Input: part model. Units: mm. Frame: model coordinates. A direction names the side the tool comes from. Round coordinates to 2 decimals unless told otherwise and drop trailing zeros. Loops run counter-clockwise (first coordinate to the right, second up) from the corner with the lowest first, then second, coordinate; pieces in that order, holes last.
1) Draft query along X for faces 1 (the face through (25, -26, 3)), 2 (the face through (-0.54, 52.33, 2.54)), 3 (the face through (0, -100, 20)). Return one class per face: pulls with the +X half, pulls with the -X half, needs draft (parallel to the pull), parting line crosses it, or undercut.
2) Section B-B, the plane y = 54.77. Return loops of the section in (x, z), and give its area (3 significant figures).
3) Access query for faces 4 (the face through (-25, -27, 4)), 5 (the face through (0, -9, 5)). Directions: +Z, -Z, +X, -X, +Y, -Y. A direction counts if a zero-diameter tool reaches every point of the face in a straight line with its end or side. Return the directions, or none.
4) Section D-D, the plane x = -19. Return loops of the section in (y, z).
5) First-contact query: pin 1 (9 mm diameter, centred on x = -8.5, z = 14.5, fed in from +Y); pin 2 (25 mm diameter, centred on x = -3, y = -45.5, fed in from +Z). Flat tips, straight axial feed; report the tip coordinate or a pass-through.
6) Section A-A, the plane x = 0. Return loops of the section in (y, z).
7) Ray query, line 1 along Y through (x, z) = (0, 3); line 2 along X through (y, z) = (42.6, 1.2); line 3 along Z through (x, y) = (-2, -86.5). Return the intervals inside material, ascending.
8) Section C-C, the plane z = 9. Return loops of the section in (x, y).
Autodesk Inventor part; units mm, degrees
ref_plane "YZ Plane" through (0, 0, 0) normal (1, 0, 0) x (0, 1, 0)
ref_plane "XZ Plane" through (0, 0, 0) normal (0, 1, 0) x (-1, 0, 0)
ref_plane "XY Plane" through (0, 0, 0) normal (0, 0, 1) x (1, 0, 0)
sketch "Sketch1" plane through (0, 0, 0) normal (0, 0, 1) x (1, 0, 0)
  line L0 (-25, -110) -> (-25, 110)
  line L1 (-25, 110) -> (25, 110)
  line L2 (25, 110) -> (25, -110)
  line L3 (25, -110) -> (-25, -110)
  line L4 (-25, -110) -> (25, 110) construction
  line L5 (-25, 110) -> (25, -110) construction
  line L6 (-25, -110) -> (-25, -105)
  line L7 (-25, -105) -> (25, -105)
  point P0 (0, 0)
  dimension "d0" = 220
  dimension "d1" = 50
  dimension "d2" = 5
extrude "Extrusion1" add sketch "Sketch1" along normal blind 5 contours L0 L1 L2 L7
sketch "Sketch2" plane through (0, 0, 5) normal (0, 0, 1) x (1, 0, 0)
  line L0 (-25, 110) -> (-25, -105)
  line L1 (-25, -105) -> (-25, -100)
  line L2 (-25, -100) -> (25, -100)
  line L3 (25, -105) -> (25, 110)
  line L4 (25, -100) -> (25, -105)
  line L5 (-25, -105) -> (25, -105)
  line L6 (-25, -105) -> (25, -105)
  point P0 (0, 0)
  dimension "d5" = 5
extrude "Extrusion2" add sketch "Sketch2" along normal blind 30
sketch "Sketch3" plane through (0, 0, 5) normal (0, 0, 1) x (1, 0, 0)
  line L0 (25, 110) -> (-25, 110)
  line L1 (0, 110) -> (-5, 110)
  line L2 (-5, 110) -> (5, 110)
  arc A0 (-5, 110) -> (5, 110) centre (0, 110) ccw
  point P0 (0, 0)
  dimension "d8" = 5
  dimension "d9" = 10
  dimension "d10" = 5
extrude "Extrusion3" cut sketch "Sketch3" against normal blind 30
ref_plane "Work Plane1" through (0, -105, 0) normal (1, 0, 0) x (0, 0, -1)
sketch "Sketch4" plane through (25, 110, 5) normal (0, 1, 0) x (1, 0, 0)
  line L0 (0, 0) -> (0, -30)
  line L1 (-50, 5) -> (-50, -30)
  line L2 (0, 0) -> (-50, 0)
  line L3 (-50, 0) -> (-50, 5)
  line L4 (-50, 5) -> (0, 5)
  line L5 (0, 5) -> (0, 0)
  point P0 (-25, 5)
extrude "Extrusion4" cut sketch "Sketch4" against normal blind 30
sketch "Sketch5" plane through (0, 0, 5) normal (0, 0, 1) x (1, 0, 0)
  line L0 (-25, 80) -> (25, 80)
  line L1 (0, 80) -> (-10, 80)
  line L2 (-10, 80) -> (10, 80)
  arc A0 (-10, 80) -> (10, 80) centre (0, 80) ccw
  point P0 (0, 0)
  dimension "d15" = 10
  dimension "d16" = 20
  dimension "d17" = 10
extrude "Extrusion5" cut sketch "Sketch5" against normal blind 30
sketch "Sketch6" plane through (0, 0, 5) normal (0, 0, 1) x (1, 0, 0)
  line L0 (0, 80) -> (0, 54.77)
  line L1 (0, 54.77) -> (0, 42.6)
  circle A0 centre (0, 54.77) radius 2.5
  circle A1 centre (0, 42.6) radius 2.5
  point P0 (0, 0)
  dimension "d20" = 25.23
  dimension "d21" = 12.17
  dimension "d22" = 5
  dimension "d23" = 5
extrude "Extrusion6" cut sketch "Sketch6" against normal blind 30
sketch "Sketch7" plane through (0, 0, 5) normal (0, 0, 1) x (1, 0, 0)
  arc A0 (-10, 80) -> (10, 80) centre (0, 80) ccw
  line L0 (10, 80) -> (25, 80)
  arc A1 (-10, 80) -> (10, 80) centre (0, 76.3471) ccw
  point P0 (0, 0)
extrude "Extrusion7" cut sketch "Sketch7" against normal blind 30
properties part number "Large Syring Mount"
Final values:
1. face 1: pulls with the +X half
1. face 2: undercut
1. face 3: needs draft
2. outline: (-25, 0) - (-2.5, 0) - (-2.5, 5) - (-25, 5) - close; (2.5, 0) - (25, 0) - (25, 5) - (2.5, 5) - close
2. area: 225 mm2
3. face 4: +Z, -Z, -X, +Y, -Y
3. face 5: +Z, +X, -X, +Y
4. outline: (-105, 0) - (80, 0) - (80, 5) - (-100, 5) - (-100, 35) - (-105, 35) - close
5. pin 1: stops at y = -100
5. pin 2: stops at z = 5
6. outline: (-105, 0) - (40.1, 0) - (40.1, 5) - (-100, 5) - (-100, 35) - (-105, 35) - close; (45.1, 0) - (52.27, 0) - (52.27, 5) - (45.1, 5) - close; (57.27, 0) - (65.7, 0) - (65.7, 5) - (57.27, 5) - close
7. line 1: y = -105 to 40.1, 45.1 to 52.27, 57.27 to 65.7
7. line 2: x = -25 to -2.5, 2.5 to 25
7. line 3: z = 0 to 5
8. outline: (-25, -105) - (25, -105) - (25, -100) - (-25, -100) - close
